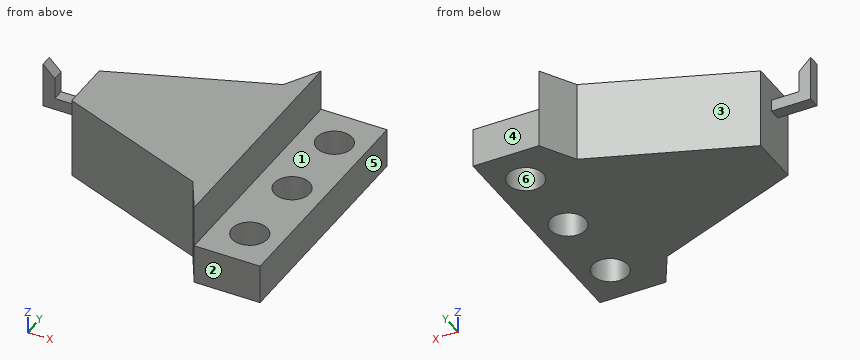
```python
from build123d import *

# Parameters (mm, degrees)
SKETCH1_W                = 8.509
SKETCH1_H                = 30.48
SKETCH1_R                = 2.286
BOSS_EXTRUDE1_DEPTH      = 5.08
BOSS_EXTRUDE2_DEPTH      = 10.414
BOSS_EXTRUDE3_DEPTH      = 0.762
BOSS_EXTRUDE3_DEPTH_BACK = 0.762


with BuildPart() as part:
    # Sketch1 → Boss-Extrude1 (new body)
    with BuildSketch(Plane.XY):
        with Locations((-4.2545, -15.24)):
            Rectangle(SKETCH1_W, SKETCH1_H)
        with Locations((-4.064, -15.24)):
            Circle(SKETCH1_R, mode=Mode.SUBTRACT)
        with Locations((-4.064, -25.4)):
            Circle(SKETCH1_R, mode=Mode.SUBTRACT)
        with Locations((-4.064, -5.08)):
            Circle(SKETCH1_R, mode=Mode.SUBTRACT)
    extrude(amount=BOSS_EXTRUDE1_DEPTH)

    # Sketch1_3 → Boss-Extrude2 (add)
    with BuildSketch(Plane.XY):
        Polygon((-8.509, 0), (-8.509, -30.48), (-11.049, -26.080590949), (-30.734, -18.542), (-30.734, -11.938), (-11.049, -4.399409051), align=None)
    extrude(amount=BOSS_EXTRUDE2_DEPTH)

    # Sketch2 → Boss-Extrude3 (add, two sides: drawn at the far end of the back side and taken through both)
    with BuildSketch(Plane(origin=(0, -15.24, 0), x_dir=(-1, 0, 0), z_dir=(0, -1, 0)).offset(-BOSS_EXTRUDE3_DEPTH_BACK)):
        Polygon((35.814, -6.39), (30.734, -6.39), (30.734, -7.914), (34.29, -7.914), (34.29, -10.668), (35.814, -12.192), align=None)
    extrude(amount=BOSS_EXTRUDE3_DEPTH + BOSS_EXTRUDE3_DEPTH_BACK)


solid = part.part
```
Here's how the part is built. I have some questions about the finished solid (model axes, mm). Face numbers are marked on the shaded views. A direction names the side the tool comes from. Give positions to 0.01 mm unless a question says otherwise; leave off trailing zeros. Loops run counter-clockwise (first coordinate to the right, second up) from the corner with the lowest first, then second, coordinate; pieces in that order, holes last. Notation, with made-up numbers: M -10.5,2.25 L 10.5,2.25 A38 ccw 10.5,41.25 Z; hole C 51.5,-22 d2. An arc over 180 degrees is marked long. Put each result on its own line as item: value. Start each with the question number.
(1) If we mould it in two halves opening along X, with no side actions, what happens to the marked faces 3, 4, 5 and 6? For each: +X half, -X half, draft (parallel to the pull), parting line (faces both ways), or undercut.
(2) I want a section at D-D on y = -25.4. Please give me the cut outline in (x, z).
(3) For the marked faces 1 and 2, which set-ups out of +Z, -Z, +X, -X, +Y, -Y let a thin tool reach every point of the face, with its end or its side?
(4) I want a section at C-C on z = 1. Please give me the cut outline in (x, y), then the cut area to 3 significant figures.
(5) Will these pins go through, and if not, where does the flat tip stop? pin 1 Ø7.5 at (x, y) = (-4.064, -25.4) entering from +Z; pin 2 Ø4 at (x, z) = (-33.5, 8.5) entering from +Y; pin 3 Ø2 at (y, z) = (-19.5, 5) entering from -X.
(6) I need wall thicknesses on line 1 along Z through (x, y) = (-25.5, -19.5); line 2 along Z through (x, y) = (-1.5, -7.5); line 3 along X through (y, z) = (-18, 3.75). Which ranges of each line are inside material? Lowest first, please. Write a range as [from, to].
(7) I want a section at A-A on y = -15.24. Please give me the cut outline in (x, z), then the cut area to 3 significant figures.
(8) I want a section at B-B on z = 10. Please give me the cut outline in (x, y), then the cut area to 3 significant figures.
Answer block:
1. face 3: -X half
1. face 4: draft
1. face 5: +X half
1. face 6: undercut
2. outline: M -12.83,0 L -6.35,0 L -6.35,5.08 L -8.51,5.08 L -8.51,10.41 L -12.83,10.41 Z; M -1.78,0 L 0,0 L 0,5.08 L -1.78,5.08 Z
3. face 1: +Z, +X, +Y, -Y
3. face 2: +Z, -Z, +X, -X, -Y
4. outline: M -30.73,-18.54 L -11.05,-26.08 L -8.51,-30.48 L 0,-30.48 L 0,0 L -8.51,0 L -11.05,-4.4 L -30.73,-11.94 Z; hole C -4.06,-25.4 d4.57; hole C -4.06,-15.24 d4.57; hole C -4.06,-5.08 d4.57
4. area: 555 mm^2
5. pin 1: z = 5.08
5. pin 2: y = -14.48
5. pin 3: x = -30.73
6. line 1: [0, 10.41]
6. line 2: [0, 5.08]
6. line 3: [-30.73, 0]
7. outline: M -35.81,6.39 L -30.73,6.39 L -30.73,0 L -6.35,0 L -6.35,5.08 L -8.51,5.08 L -8.51,10.41 L -30.73,10.41 L -30.73,7.91 L -34.29,7.91 L -34.29,10.67 L -35.81,12.19 Z; M -1.78,0 L 0,0 L 0,5.08 L -1.78,5.08 Z
7. area: 265 mm^2
8. outline: M -35.81,-16 L -34.29,-16 L -34.29,-14.48 L -35.81,-14.48 Z; M -30.73,-18.54 L -11.05,-26.08 L -8.51,-30.48 L -8.51,0 L -11.05,-4.4 L -30.73,-11.94 Z
8. area: 347 mm^2
